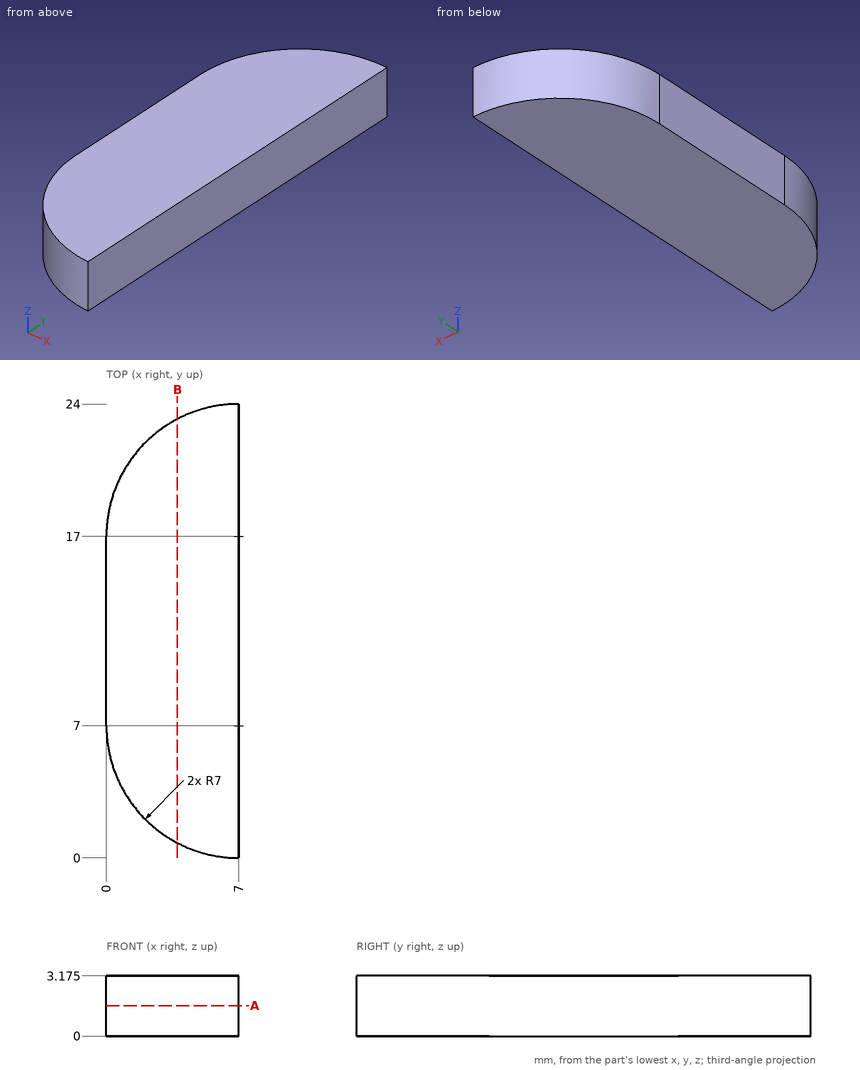
Print and shaded views of the part. All mm, measured from the part's lowest x, y and z. Coordinates: 2 decimals unless noted, no trailing zeros. Loops run counter-clockwise (first coordinate to the right, second up) from the corner with the lowest first, then second, coordinate; pieces in that order, holes last. Notation, with made-up numbers: (-27, 51.25) - (-11, 51.25) arc R16 cw to (-11, 58.25) - close; hole circle Ø11 at (65.5, 16). An arc over 180 degrees is marked (long way). Write item = value, one per line. Start each with the question number.
Item 1: Saw through at A-A, the plane z = 1.6. List the corners of the cut face in (x, y), then the cut area to 3 significant figures.
Item 2: Drop a flat-ended pin along its axis: pin 1 Ø1 at (x, z) = (3, 1) entering from -Y. Give the stop position or say it passes through.
Item 3: Wall check: probe 1 along Y at (x, z) = (6.75, 1.25); probe 2 along Y at (x, z) = (1.25, 0.95); probe 3 along X at (y, z) = (4.25, 1.75). Give the ranges that are in metal, low to high. Write a range as [from, to].
Item 4: Saw through at B-B, the plane x = 3.75. List the corners of the cut face in (y, z) (3 decimals).
Answers:
q1.outline = (0, 7) arc R7 ccw to (7, 0) - (7, 24) arc R7 ccw to (0, 17) - close
q1.area = 147 mm2
q2.pin_1 = 0.94
q3.probe_1 = [0, 24]
q3.probe_2 = [3.01, 20.99]
q3.probe_3 = [0.56, 7]
q4.outline = (0.8, 0) - (23.2, 0) - (23.2, 3.175) - (0.8, 3.175) - close
